from build123d import *

# Parameters (mm, degrees)
F0_W     = 76.2
F0_H     = 123.29414
F0_W_2   = 68.58
F0_H_2   = 115.67414
F1_DEPTH = 3.81
F0_W_3   = 60.96
F0_H_3   = 108.05414
F2_DEPTH = 7.62
F0_W_4   = 53.34
F0_H_4   = 100.43414
F3_DEPTH = 11.43
F4_DEPTH = 15.24
F5_R     = 2.54
F6_DEPTH = 25.4


with BuildPart() as f1:
    # F0 (on Top) → F1 (new body)
    with BuildSketch(Plane.XY):
        Rectangle(F0_W, F0_H)
        Rectangle(F0_W_2, F0_H_2, mode=Mode.SUBTRACT)
    extrude(amount=F1_DEPTH)

    # F0 (on Top) → F2 (join)
    with BuildSketch(Plane.XY):
        Rectangle(F0_W_2, F0_H_2)
        Rectangle(F0_W_3, F0_H_3, mode=Mode.SUBTRACT)
    extrude(amount=F2_DEPTH)

    # F0 (on Top) → F3 (join)
    with BuildSketch(Plane.XY):
        Rectangle(F0_W_3, F0_H_3)
        Rectangle(F0_W_4, F0_H_4, mode=Mode.SUBTRACT)
    extrude(amount=F3_DEPTH)

    # F0 (on Top) → F4 (join)
    with BuildSketch(Plane.XY):
        Rectangle(F0_W_4, F0_H_4)
    extrude(amount=F4_DEPTH)

    # F5 (on face) → F6 (join)
    with BuildSketch(Plane.XY.offset(15.24)):
        with Locations((-15.24, 46.40707)):
            Circle(F5_R)
        with Locations((-22.86, 46.40707)):
            Circle(F5_R)
        with Locations((-7.62, 46.40707)):
            Circle(F5_R)
        with Locations((-22.86, 37.964364)):
            Circle(F5_R)
        with Locations((-22.86, 29.531564)):
            Circle(F5_R)
        with Locations((-22.86, 21.093938)):
            Circle(F5_R)
        with Locations((-22.86, 12.656312)):
            Circle(F5_R)
        with Locations((-22.86, 4.218686)):
            Circle(F5_R)
        with Locations((-22.86, -4.21894)):
            Circle(F5_R)
        with Locations((-22.86, -12.656566)):
            Circle(F5_R)
        with Locations((7.62, 46.40707)):
            Circle(F5_R)
        with Locations((15.24, 46.40707)):
            Circle(F5_R)
        with Locations((22.86, 46.40707)):
            Circle(F5_R)
        with Locations((22.86, 37.969444)):
            Circle(F5_R)
        with Locations((22.86, 29.531818)):
            Circle(F5_R)
        with Locations((22.86, 21.094192)):
            Circle(F5_R)
        with Locations((22.86, 12.656566)):
            Circle(F5_R)
        with Locations((22.86, 4.21894)):
            Circle(F5_R)
        with Locations((22.86, -4.218686)):
            Circle(F5_R)
        with Locations((22.86, -12.656312)):
            Circle(F5_R)
        with Locations((-22.86, -21.094192)):
            Circle(F5_R)
        with Locations((-22.86, -29.531818)):
            Circle(F5_R)
        with Locations((-22.86, -37.969444)):
            Circle(F5_R)
        with Locations((-22.86, -46.40707)):
            Circle(F5_R)
        with Locations((-15.24, -46.40707)):
            Circle(F5_R)
        with Locations((-7.62, -46.40707)):
            Circle(F5_R)
        with Locations((7.62, -46.40707)):
            Circle(F5_R)
        with Locations((15.24, -46.40707)):
            Circle(F5_R)
        with Locations((22.86, -46.40707)):
            Circle(F5_R)
        with Locations((22.86, -37.96919)):
            Circle(F5_R)
        with Locations((22.86, -29.531564)):
            Circle(F5_R)
        with Locations((22.86, -21.093938)):
            Circle(F5_R)
    extrude(amount=F6_DEPTH)


solid = f1.part
Geometry check sheet. Reference: the model listing, model coordinates, mm. A direction names the side the tool comes from. Give positions to 0.01 mm unless a question says otherwise; leave off trailing zeros. Loops run counter-clockwise (first coordinate to the right, second up) from the corner with the lowest first, then second, coordinate; pieces in that order, holes last. Notation, with made-up numbers: M -24.75,53 L -5.75,53 A14 cw -5.75,79 Z; hole C 19.25,12.25 d8. An arc over 180 degrees is marked long. Answer as a JSON object with one key per item and string values. Group by question number.
Item 1: Access from +Z, -Z, +X, -X, +Y, -Y to the whole of each face (thin tool, end or side, straight path). Record for faces 4 (the cylindrical face through (-12.817, 47.17, 27.762)), 5 (the flat face through (23, -21, 40.64)), 6 (the flat face through (-26.67, -1, 13)).
Item 2: Gauge pin test, flat ends, axial feed: pin 1 (8 mm diameter, centred on x = -7, y = -1, fed in from +Z); pin 2 (4 mm diameter, centred on y = 20, z = 9, fed in from -X); pin 3 (3 mm diameter, centred on x = -6, z = 12.5, fed in from +Y); pin 4 (4 mm diameter, centred on x = -2, z = 5.5, fed in from +Y). Record the tip position at first contact, or that the pin passes through.
Item 3: Sectioned sample at C-C on y = 33.5. Record the boundary of the cut face in (x, z), plus the area to 3 significant figures.
Item 4: Sectioned sample at A-A on z = 18.5. Give the number of separate pieces and of enclosed holes in the cut face, plus the area to 3 significant figures.
Item 5: Mould release check, pull along Y, two halves, no side actions. Record for faces 1 (the cylindrical face through (-20.514, 20.121, 27.762)), 2 (the flat face through (-23, -38, 40.64)), 3 (the flat face through (0, -50.217, 13)): pulls with the +Y half, pulls with the -Y half, needs draft (parallel to the pull), parting line crosses it, or undercut.
Item 6: Material ranges on L1, parallel to X at y = 46, z = 36; L2, parallel to Y at x = 15, z = 33; L3, parallel to X at y = 31, z = 9, recorded low to high.
Item 7: Sectioned sample at B-B on x = 7.62. Record the boundary of the cut face in (y, z).
Item 8: Sectioned sample at D-D on z = 6. Record the boundary of the cut face in (x, y), plus the area to 3 significant figures.
Findings below:
{
 "1": {"face 4": "+Z", "face 5": "+Z, +X, -X, +Y, -Y", "face 6": "+Z, -X, +Y, -Y"},
 "2": {"pin 1": "z = 15.24", "pin 2": "x = -34.29", "pin 3": "y = 54.03", "pin 4": "y = 61.65"},
 "3": {"outline": "M -38.1,0 L 38.1,0 L 38.1,3.81 L 34.29,3.81 L 34.29,7.62 L 30.48,7.62 L 30.48,11.43 L 26.67,11.43 L 26.67,15.24 L -26.67,15.24 L -26.67,11.43 L -30.48,11.43 L -30.48,7.62 L -34.29,7.62 L -34.29,3.81 L -38.1,3.81 Z", "area": "987 mm2"},
 "4": {"separate pieces": "32", "enclosed holes": "0", "area": "649 mm2"},
 "5": {"face 1": "undercut", "face 2": "needs draft", "face 3": "pulls with the -Y half"},
 "6": {"L1": "-25.37 to -20.35, -17.75 to -12.73, -10.13 to -5.11, 5.11 to 10.13, 12.73 to 17.75, 20.35 to 25.37", "L2": "-48.94 to -43.88, 43.88 to 48.94", "L3": "-30.48 to 30.48"},
 "7": {"outline": "M -61.65,0 L 61.65,0 L 61.65,3.81 L 57.84,3.81 L 57.84,7.62 L 54.03,7.62 L 54.03,11.43 L 50.22,11.43 L 50.22,15.24 L 48.95,15.24 L 48.95,40.64 L 43.87,40.64 L 43.87,15.24 L -43.87,15.24 L -43.87,40.64 L -48.95,40.64 L -48.95,15.24 L -50.22,15.24 L -50.22,11.43 L -54.03,11.43 L -54.03,7.62 L -57.84,7.62 L -57.84,3.81 L -61.65,3.81 Z"},
 "8": {"outline": "M -34.29,-57.84 L 34.29,-57.84 L 34.29,57.84 L -34.29,57.84 Z", "area": "7,930 mm2"}
}
